Geometry: final body of the model. Coordinates: model frame, mm. A direction names the side the tool comes from. Give positions to 0.01 mm unless a question says otherwise; leave off trailing zeros. Loops run counter-clockwise (first coordinate to the right, second up) from the corner with the lowest first, then second, coordinate; pieces in that order, holes last.
from build123d import *

# Parameters (mm, degrees)
F2_R     = 1.5
F3_DEPTH = 5
F4_R     = 1.5
F5_DEPTH = 5


with BuildPart() as f1:
    # F0 (on Right) → F1 (revolve)
    with BuildSketch(Plane.YZ):
        Polygon((-20, 2.5), (-20, 0), (50, 0), (50, 6), (46.5, 6), (46.5, 12.7), (40, 21.25), (4.4, 21.25), (0, 18.4), (0, 2.5), align=None)
    revolve(axis=Axis((0, 15, 0), (0, -1, 0)))

    # F2 (on face) → F3 (cut)
    with BuildSketch(Plane.XZ):
        with Locations((12.5, 0)):
            Circle(F2_R)
        with Locations((0, 12.5)):
            Circle(F2_R)
        with Locations((-12.5, 0)):
            Circle(F2_R)
        with Locations((0, -12.5)):
            Circle(F2_R)
    extrude(amount=-F3_DEPTH, mode=Mode.SUBTRACT)

    # F4 (on face) → F5 (cut)
    with BuildSketch(Plane(origin=(0, 46.5, 0), x_dir=(-1, 0, 0), z_dir=(0, 1, 0))):
        with Locations((8.5, 0)):
            Circle(F4_R)
        with Locations((0, 8.5)):
            Circle(F4_R)
        with Locations((-8.5, 0)):
            Circle(F4_R)
        with Locations((0, -8.5)):
            Circle(F4_R)
    extrude(amount=-F5_DEPTH, mode=Mode.SUBTRACT)


solid = f1.part
Item 1: Ray query, probe 1 along Z at (x, y) = (0, 43.05); probe 2 along Y at (x, z) = (-0.5, -10); probe 3 along Y at (x, z) = (1, 5). Return the intervals inside material, ascending.
Values follow:
probe 1: z = -17.24 to -10, -7 to 7, 10 to 17.24
probe 2: y = 0 to 46.5
probe 3: y = 0 to 50
Item 2: Section query C-C on y = -2.5. Return loops of the section in (x, z), plus the area to 3 significant figures.
Values follow:
outline: circle Ø5 at (0, 0)
area: 19.6 mm2
Item 3: Pin query (flat end, axial travel): pin 1 (12 mm diameter, centred on x = 1, z = -14.5, fed in from -Y); pin 2 (2.5 mm diameter, centred on x = 0, z = 8.5, fed in from +Y); pin 3 (12 mm diameter, centred on x = -10, z = -4, fed in from +Y); pin 4 (4 mm diameter, centred on x = -9.5, y = 17, fed in from +Z). Return the tip coordinate at first contact, or that it passes through.
Values follow:
pin 1: stops at y = 0
pin 2: stops at y = 41.5
pin 3: stops at y = 50
pin 4: stops at z = 19.88
Item 4: Draft query along X for faces 1 (the face through (0, 44, -10)), 2 (the face through (0, 48, -6)), 3 (the face through (0, 5, 13)), 4 (the face through (0, -20, 0)). Return one class per face: +X half, -X half, draft (parallel to the pull), parting line (faces both ways), or undercut.
Values follow:
face 1: undercut
face 2: parting line
face 3: undercut
face 4: draft
Item 5: Set-up query: faces 5 (the face through (0, 50, 0)), 6 (the face through (0, 41.5, 9)), 7 (the face through (12, 5, 0)). Return all of +Z, -Z, +X, -X, +Y, -Y with unobstructed straight access to the full face (end or side cutting, diameter ignored); none if empty.
Values follow:
face 5: +Z, -Z, +X, -X, +Y
face 6: +Y
face 7: -Y
Item 6: Section query B-B on y = 24. Return loops of the section in (x, z), plus the area to 3 significant figures.
Values follow:
outline: circle Ø42.5 at (0, 0)
area: 1,420 mm2
